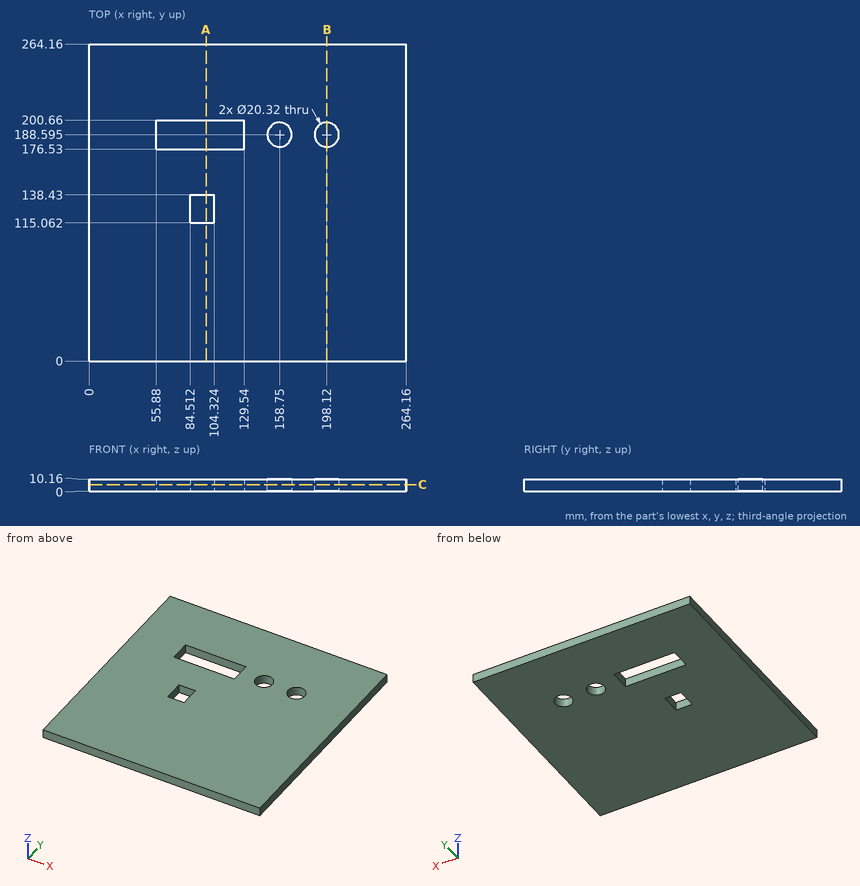
The drawing under review shows one solid part. Ordinate dimensions are in mm from its lowest x, y, z. Coordinates: 2 decimals unless noted, no trailing zeros. Order: outer loops, then holes, each group sorted by start corner. A loop starts at its lowest first (then second) coordinate and runs counter-clockwise, first axis right, second up. Notation, with made-up numbers: (32, -8.5) - (85, -8.5) arc R25 cw to (85, 3.5) - close; hole circle Ø5 at (28, -12.75). An arc over 180 degrees is marked (long way). Put each result on its own line as item: value.
1) Wall thickness on L1, parallel to Y at x = 198.12, z = 3.75 (1 decimal); L2, parallel to Y at x = 91.5, z = 8.75; L3, parallel to Y at x = 166, z = 9.25 (1 decimal): over which ranges is each line inside the solid? List them lowest first. Write a range as from..to.
Response values:
L1: y = 0..178.4, 198.8..264.2
L2: y = 0..115.06, 138.43..176.53, 200.66..264.16
L3: y = 0..181.5, 195.7..264.2
2) Take a section at A-A, the plane x = 97.5. Give the boundary of the cut face in (y, z).
Response values:
outline: (0, 0) - (115.06, 0) - (115.06, 10.16) - (0, 10.16) - close; (138.43, 0) - (176.53, 0) - (176.53, 10.16) - (138.43, 10.16) - close; (200.66, 0) - (264.16, 0) - (264.16, 10.16) - (200.66, 10.16) - close
3) Take a section at B-B, the plane x = 198.12. Give the boundary of the cut face in (y, z) (1 decimal).
Response values:
outline: (0, 0) - (178.4, 0) - (178.4, 10.2) - (0, 10.2) - close; (198.8, 0) - (264.2, 0) - (264.2, 10.2) - (198.8, 10.2) - close
4) Take a section at C-C, the plane z = 5.5. Count the separate pieces of the cut face and the enclosed holes in it, and give its area (3 significant figures).
Response values:
separate pieces: 1
enclosed holes: 4
area: 66,900 mm²
